For this review, take the finished solid that the model builds, in its own axes (mm). Round coordinates to 2 decimals unless told otherwise and drop trailing zeros. Order: outer loops, then holes, each group sorted by start corner. A loop starts at its lowest first (then second) coordinate and runs counter-clockwise, first axis right, second up. Notation, with made-up numbers: M -7,39 L 43,39 A14 cw 43,53 Z; hole C 63.5,5 d6. An arc over 180 degrees is marked long. Use a Markdown table: item, result.
from build123d import *

# Parameters (mm, degrees)
SKETCH1_R           = 1.5
BOSS_EXTRUDE1_DEPTH = 2.6
BOSS_EXTRUDE2_START = -2.6
SKETCH2_R           = 1.5
BOSS_EXTRUDE2_DEPTH = 2.6
SKETCH3_R           = 1.5
SKETCH3_R_2         = 11
CUT_EXTRUDE2_DEPTH  = 2.6
SKETCH4_R           = 1.5
BOSS_EXTRUDE3_DEPTH = 2.6
BOSS_EXTRUDE5_START = -2.6
SKETCH5_R           = 1
BOSS_EXTRUDE5_DEPTH = 2.6
FILLET1_R           = 5


with BuildPart() as part:
    # Sketch1 → Boss-Extrude1 (new body)
    with BuildSketch(Plane(origin=(0, 0, 0), x_dir=(1, 0, 0), z_dir=(0, 1, 0))):
        with BuildLine():
            ThreePointArc((168.347792712, 1300.859692621), (159.343486253, 1295.942873675), (149.343647654, 1293.65030495))
            ThreePointArc((149.343647654, 1293.65030495), (139.460555114, 1295.990018463), (130.567766275, 1300.895941835))
            ThreePointArc((130.567766275, 1300.895941835), (124.616810573, 1297.0492589), (123.648598599, 1290.029756856))
            Line((123.648598599, 1290.029756856), (131.000501903, 1282.677853551))
            ThreePointArc((131.000501903, 1282.677853551), (132.734683914, 1280.082466761), (133.343647654, 1277.020999302))
            Line((133.343647654, 1277.020999302), (133.343647654, 1272.65030495))
            Line((133.343647654, 1272.65030495), (133.343647654, 1269.65030495))
            Line((133.343647654, 1269.65030495), (133.343647654, 1240.65030495))
            Line((133.343647654, 1240.65030495), (133.343647654, 1237.65030495))
            Line((133.343647654, 1237.65030495), (133.343647654, 1233.279610599))
            ThreePointArc((133.343647654, 1233.279610599), (132.734683914, 1230.21814314), (131.000501903, 1227.622756349))
            Line((131.000501903, 1227.622756349), (123.648598599, 1220.270853045))
            ThreePointArc((123.648598599, 1220.270853045), (124.616810573, 1213.251351001), (130.567766275, 1209.404668065))
            ThreePointArc((130.567766275, 1209.404668065), (139.460555114, 1214.310591438), (149.343647654, 1216.65030495))
            ThreePointArc((149.343647654, 1216.65030495), (159.343486253, 1214.357736226), (168.347792712, 1209.44091728))
            ThreePointArc((168.347792712, 1209.44091728), (174.131892083, 1213.349250607), (175.038696709, 1220.270853045))
            Line((175.038696709, 1220.270853045), (167.686793404, 1227.622756349))
            ThreePointArc((167.686793404, 1227.622756349), (165.952611394, 1230.21814314), (165.343647654, 1233.279610599))
            Line((165.343647654, 1233.279610599), (165.343647654, 1237.65030495))
            Line((165.343647654, 1237.65030495), (165.343647654, 1240.65030495))
            Line((165.343647654, 1240.65030495), (165.343647654, 1269.65030495))
            Line((165.343647654, 1269.65030495), (165.343647654, 1272.65030495))
            Line((165.343647654, 1272.65030495), (165.343647654, 1277.020999302))
            ThreePointArc((165.343647654, 1277.020999302), (165.952611394, 1280.082466761), (167.686793404, 1282.677853551))
            Line((167.686793404, 1282.677853551), (175.038696709, 1290.029756856))
            ThreePointArc((175.038696709, 1290.029756856), (174.131892083, 1296.951359294), (168.347792712, 1300.859692621))
        make_face()
        with Locations(Location((130.843647654, 1216.65030495, 0), (0, 0, 270))):
            Circle(SKETCH1_R, mode=Mode.SUBTRACT)
        with Locations(Location((149.343647654, 1222.919184261, 0), (0, 0, 270))):
            Circle(SKETCH1_R, mode=Mode.SUBTRACT)
        with Locations(Location((167.843647654, 1216.65030495, 0), (0, 0, 270))):
            Circle(SKETCH1_R, mode=Mode.SUBTRACT)
        with Locations(Location((130.843647654, 1293.65030495, 0), (0, 0, 270))):
            Circle(SKETCH1_R, mode=Mode.SUBTRACT)
        with Locations(Location((149.343647654, 1287.38142564, 0), (0, 0, 270))):
            Circle(SKETCH1_R, mode=Mode.SUBTRACT)
        with BuildLine():
            ThreePointArc((169.343647654, 1293.65030495), (167.843647654, 1292.15030495), (166.343647654, 1293.65030495))
            ThreePointArc((166.343647654, 1293.65030495), (167.843647654, 1295.15030495), (169.343647654, 1293.65030495))
        make_face(mode=Mode.SUBTRACT)
    extrude(amount=BOSS_EXTRUDE1_DEPTH)

    # Sketch2 → Boss-Extrude2 (add)
    # profile 1 of 4: a face of its own
    with BuildSketch(Plane(origin=(0, 2.6, 0), x_dir=(1, 0, 0), z_dir=(0, 1, 0)).offset(BOSS_EXTRUDE2_START)):
        with BuildLine():
            Line((171.362745056, 1223.946804697), (172.733437461, 1229.278912352))
            ThreePointArc((172.733437461, 1229.278912352), (172.109499611, 1232.295080685), (169.343647654, 1233.65030495))
            Line((169.343647654, 1233.65030495), (165.343647654, 1233.279610599))
            ThreePointArc((165.343647654, 1233.279610599), (165.952611394, 1230.21814314), (167.686793404, 1227.622756349))
            Line((167.686793404, 1227.622756349), (171.362745056, 1223.946804697))
        make_face()
        with Locations(Location((169.343647654, 1230.15030495, 0), (0, 0, 270))):
            Circle(SKETCH2_R, mode=Mode.SUBTRACT)
    # profile 2 of 4: a face of its own
    with BuildSketch(Plane(origin=(0, 2.6, 0), x_dir=(1, 0, 0), z_dir=(0, 1, 0)).offset(BOSS_EXTRUDE2_START)):
        with BuildLine():
            Line((127.324550251, 1223.946804697), (131.000501903, 1227.622756349))
            ThreePointArc((131.000501903, 1227.622756349), (132.734683914, 1230.21814314), (133.343647654, 1233.279610599))
            Line((133.343647654, 1233.279610599), (129.343647654, 1233.65030495))
            ThreePointArc((129.343647654, 1233.65030495), (126.577795697, 1232.295080685), (125.953857846, 1229.278912352))
            Line((125.953857846, 1229.278912352), (127.324550251, 1223.946804697))
        make_face()
        with Locations(Location((129.343647654, 1230.15030495, 0), (0, 0, 270))):
            Circle(SKETCH2_R, mode=Mode.SUBTRACT)
    # profile 3 of 4: a face of its own
    with BuildSketch(Plane(origin=(0, 2.6, 0), x_dir=(1, 0, 0), z_dir=(0, 1, 0)).offset(BOSS_EXTRUDE2_START)):
        with BuildLine():
            Line((171.362745056, 1286.353805203), (172.733437461, 1281.021697549))
            ThreePointArc((172.733437461, 1281.021697549), (172.109499611, 1278.005529215), (169.343647654, 1276.65030495))
            Line((169.343647654, 1276.65030495), (165.343647654, 1277.020999302))
            ThreePointArc((165.343647654, 1277.020999302), (165.952611394, 1280.082466761), (167.686793404, 1282.677853551))
            Line((167.686793404, 1282.677853551), (171.362745056, 1286.353805203))
        make_face()
        with Locations(Location((169.343647654, 1280.15030495, 0), (0, 0, 270))):
            Circle(SKETCH2_R, mode=Mode.SUBTRACT)
    # profile 4 of 4: a face of its own
    with BuildSketch(Plane(origin=(0, 2.6, 0), x_dir=(1, 0, 0), z_dir=(0, 1, 0)).offset(BOSS_EXTRUDE2_START)):
        with BuildLine():
            Line((127.324550251, 1286.353805203), (125.953857846, 1281.021697549))
            ThreePointArc((125.953857846, 1281.021697549), (126.577795697, 1278.005529215), (129.343647654, 1276.65030495))
            Line((129.343647654, 1276.65030495), (133.343647654, 1277.020999302))
            ThreePointArc((133.343647654, 1277.020999302), (132.734683914, 1280.082466761), (131.000501903, 1282.677853551))
            Line((131.000501903, 1282.677853551), (127.324550251, 1286.353805203))
        make_face()
        with Locations(Location((129.343647654, 1280.15030495, 0), (0, 0, 270))):
            Circle(SKETCH2_R, mode=Mode.SUBTRACT)
    extrude(amount=BOSS_EXTRUDE2_DEPTH)

    # Sketch3 → Cut-Extrude2 (cut)
    with BuildSketch(Plane(origin=(0, 2.6, 0), x_dir=(1, 0, 0), z_dir=(0, 1, 0))):
        with Locations((134.093647654, 1239.90030495)):
            Circle(SKETCH3_R)
        with Locations((164.593647654, 1239.90030495)):
            Circle(SKETCH3_R)
        with Locations((164.593647654, 1270.40030495)):
            Circle(SKETCH3_R)
        with Locations((134.093647654, 1270.40030495)):
            Circle(SKETCH3_R)
        with Locations((169.343647654, 1255.15030495)):
            Circle(SKETCH3_R_2)
        with Locations((129.343647654, 1255.15030495)):
            Circle(SKETCH3_R_2)
    extrude(amount=-CUT_EXTRUDE2_DEPTH, mode=Mode.SUBTRACT)

    # Sketch4 → Boss-Extrude3 (add)
    # profile 1 of 4: a face of its own
    with BuildSketch(Plane(origin=(0, 2.6, 0), x_dir=(1, 0, 0), z_dir=(0, 1, 0))):
        with BuildLine():
            Line((172.677777674, 1231.215000685), (169.412849314, 1241.439232174))
            ThreePointArc((169.412849314, 1241.439232174), (160.29790956, 1242.572314655), (165.343647654, 1234.897255716))
            Line((165.343647654, 1234.897255716), (165.343647654, 1233.279610599))
            Line((165.343647654, 1233.279610599), (169.343647654, 1233.65030495))
            ThreePointArc((169.343647654, 1233.65030495), (171.408056156, 1232.976648443), (172.677777674, 1231.215000685))
        make_face()
        with Locations(Location((164.593647654, 1239.90030495, 0), (0, 0, 270))):
            Circle(SKETCH4_R, mode=Mode.SUBTRACT)
    # profile 2 of 4: a face of its own
    with BuildSketch(Plane(origin=(0, 2.6, 0), x_dir=(1, 0, 0), z_dir=(0, 1, 0))):
        with BuildLine():
            Line((129.343647654, 1233.65030495), (133.343647654, 1233.279610599))
            Line((133.343647654, 1233.279610599), (133.343647654, 1234.897255716))
            ThreePointArc((133.343647654, 1234.897255716), (138.389385748, 1242.572314655), (129.274445994, 1241.439232174))
            Line((129.274445994, 1241.439232174), (126.009517634, 1231.215000685))
            ThreePointArc((126.009517634, 1231.215000685), (127.279239152, 1232.976648443), (129.343647654, 1233.65030495))
        make_face()
        with Locations(Location((134.093647654, 1239.90030495, 0), (0, 0, 270))):
            Circle(SKETCH4_R, mode=Mode.SUBTRACT)
    # profile 3 of 4: a face of its own
    with BuildSketch(Plane(origin=(0, 2.6, 0), x_dir=(1, 0, 0), z_dir=(0, 1, 0))):
        with BuildLine():
            Line((172.677777674, 1279.085609215), (169.412849314, 1268.861377727))
            ThreePointArc((169.412849314, 1268.861377727), (160.29790956, 1267.728295245), (165.343647654, 1275.403354184))
            Line((165.343647654, 1275.403354184), (165.343647654, 1277.020999302))
            Line((165.343647654, 1277.020999302), (169.343647654, 1276.65030495))
            ThreePointArc((169.343647654, 1276.65030495), (171.408056156, 1277.323961458), (172.677777674, 1279.085609215))
        make_face()
        with Locations(Location((164.593647654, 1270.40030495, 0), (0, 0, 270))):
            Circle(SKETCH4_R, mode=Mode.SUBTRACT)
    # profile 4 of 4: a face of its own
    with BuildSketch(Plane(origin=(0, 2.6, 0), x_dir=(1, 0, 0), z_dir=(0, 1, 0))):
        with BuildLine():
            Line((126.009517634, 1279.085609215), (129.274445994, 1268.861377727))
            ThreePointArc((129.274445994, 1268.861377727), (138.389385748, 1267.728295245), (133.343647654, 1275.403354184))
            Line((133.343647654, 1275.403354184), (133.343647654, 1277.020999302))
            Line((133.343647654, 1277.020999302), (129.343647654, 1276.65030495))
            ThreePointArc((129.343647654, 1276.65030495), (127.279239152, 1277.323961458), (126.009517634, 1279.085609215))
        make_face()
        with Locations(Location((134.093647654, 1270.40030495, 0), (0, 0, 270))):
            Circle(SKETCH4_R, mode=Mode.SUBTRACT)
    extrude(amount=-BOSS_EXTRUDE3_DEPTH)

    # Sketch5 → Boss-Extrude5 (add)
    with BuildSketch(Plane(origin=(0, 2.6, 0), x_dir=(1, 0, 0), z_dir=(0, 1, 0)).offset(BOSS_EXTRUDE5_START)):
        with BuildLine():
            Line((168.347792712, 1209.44091728), (162.343647654, 1207.919184261))
            ThreePointArc((162.343647654, 1207.919184261), (159.343647654, 1204.919184261), (156.343647654, 1207.919184261))
            Line((156.343647654, 1207.919184261), (149.343647654, 1210.919184261))
            Line((149.343647654, 1210.919184261), (142.343647654, 1207.919184261))
            ThreePointArc((142.343647654, 1207.919184261), (139.343647654, 1204.919184261), (136.343647654, 1207.919184261))
            Line((136.343647654, 1207.919184261), (130.567766275, 1209.404668065))
            ThreePointArc((130.567766275, 1209.404668065), (139.460555114, 1214.310591438), (149.343647654, 1216.65030495))
            ThreePointArc((149.343647654, 1216.65030495), (159.343486253, 1214.357736226), (168.347792712, 1209.44091728))
        make_face()
        with Locations(Location((139.343647654, 1207.919184261, 0), (0, 0, 270))):
            Circle(SKETCH5_R, mode=Mode.SUBTRACT)
        with Locations(Location((159.343647654, 1207.919184261, 0), (0, 0, 270))):
            Circle(SKETCH5_R, mode=Mode.SUBTRACT)
    extrude(amount=BOSS_EXTRUDE5_DEPTH)

    # Fillet1
    fillet1_edges = [part.edges().sort_by_distance(p)[0] for p in [
        (136.343647654, 1.3, -1207.919184261),
        (142.343647654, 1.3, -1207.919184261),
        (149.343647654, 1.3, -1210.919184261),
        (156.343647654, 1.3, -1207.919184261),
        (162.343647654, 1.3, -1207.919184261),
    ]]
    fillet(fillet1_edges, radius=FILLET1_R)


solid = part.part
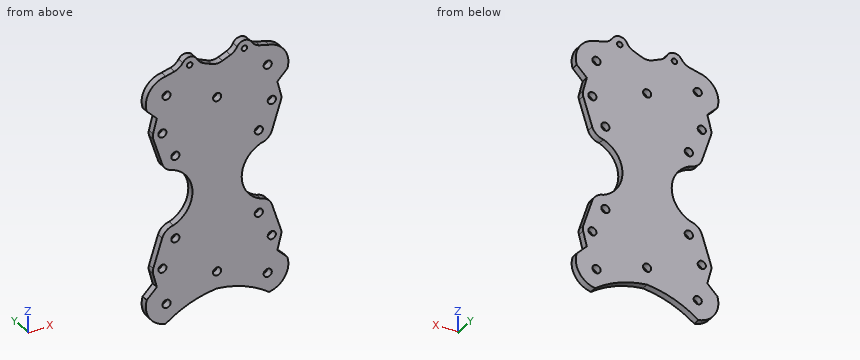
Q1. Add section B-B (y = 1.45). Give the number of separate pieces and of enclosed holes in the cut face, then the cut area to 3 significant figures.
Determined:
| item | result |
|---|---|
| separate pieces | 1 |
| enclosed holes | 16 |
| area | 3,460 mm^2 |
Q2. Add section C-C (z = -1212). Write out the cut boundary in (x, y), then the cut area to 3 significant figures.
Determined:
| item | result |
|---|---|
| outline | M 125.59,0 L 173.1,0 L 173.1,2.6 L 125.59,2.6 Z |
| area | 124 mm^2 |
Q3. Wall thickness on line 1 along Z through (x, y) = (139, 1.75); line 2 along Z through (x, y) = (168, 1.6); line 3 along Z through (x, y) = (167, 0.85): over which ranges is each line inside the solid? List them lowest first. Write a range as [from, to].
Determined:
| item | result |
|---|---|
| line 1 | z = [-1296.17, -1260.42], [-1249.88, -1208.86], [-1206.98, -1204.94] |
| line 2 | z = [-1300.61, -1295.14], [-1292.16, -1280.82], [-1279.48, -1266.66], [-1243.64, -1230.82], [-1229.48, -1218.14], [-1215.16, -1209.35] |
| line 3 | z = [-1299.91, -1294.89], [-1292.41, -1265.95], [-1244.35, -1217.89], [-1215.41, -1209.1] |
Q4. Add section A-A (z = -1264). Write out the cut boundary in (x, y).
Determined:
| item | result |
|---|---|
| outline | M 135.88,0 L 162.81,0 L 162.81,2.6 L 135.88,2.6 Z |
Q5. Clearance check with flat-ended pins moving along their axes: pin 1 (1 mm diameter, centred on y = 0.5, z = -1216.5, fed in from -X); pin 2 (1 mm diameter, centred on y = 2, z = -1238, fed in from +X); pin 3 (1 mm diameter, centred on x = 133, y = 0.5, fed in from -Z). State where each tip first meets the part, or that it passes through.
Determined:
| item | result |
|---|---|
| pin 1 | stops at x = 123.33 |
| pin 2 | stops at x = 170.67 |
| pin 3 | stops at z = -1299.55 |
